```python
from build123d import *

# Parameters (mm, degrees)
SKETCH1_W           = 156
SKETCH1_H           = 90
BOSS_EXTRUDE1_DEPTH = 3
SKETCH2_W           = 156
SKETCH2_H           = 90
SKETCH2_W_2         = 150
SKETCH2_H_2         = 84
BOSS_EXTRUDE2_DEPTH = 48
FILLET1_R           = 1
SKETCH3_W           = 12
SKETCH3_H           = 23
CUT_EXTRUDE2_DEPTH  = 157
SKETCH4_R           = 8.5
CUT_EXTRUDE3_DEPTH  = 10


with BuildPart() as part:
    # Sketch1 → Boss-Extrude1 (new body)
    with BuildSketch(Plane(origin=(0, 0, 0), x_dir=(1, 0, 0), z_dir=(0, 1, 0))):
        with Locations((78, 45)):
            Rectangle(SKETCH1_W, SKETCH1_H)
    extrude(amount=BOSS_EXTRUDE1_DEPTH)

    # Sketch2 → Boss-Extrude2 (add)
    with BuildSketch(Plane(origin=(0, 3, 0), x_dir=(1, 0, 0), z_dir=(0, 1, 0))):
        with Locations((78, 45)):
            Rectangle(SKETCH2_W, SKETCH2_H)
        with Locations((78, 45)):
            Rectangle(SKETCH2_W_2, SKETCH2_H_2, mode=Mode.SUBTRACT)
    extrude(amount=BOSS_EXTRUDE2_DEPTH)

    # Fillet1
    fillet1_edges = [part.edges().sort_by_distance(p)[0] for p in [
        (0, 25.5, -90),
        (156, 25.5, -90),
        (156, 25.5, 0),
        (0, 25.5, 0),
    ]]
    fillet(fillet1_edges, radius=FILLET1_R)

    # Sketch3 → Cut-Extrude2 (cut, through all)
    with BuildSketch(Plane(origin=(156, 0, 0), x_dir=(0, 0, -1), z_dir=(1, 0, 0))):
        with Locations((9, 14.5)):
            Rectangle(SKETCH3_W, SKETCH3_H)
        with Locations((81, 14.5)):
            Rectangle(SKETCH3_W, SKETCH3_H)
    extrude(amount=-CUT_EXTRUDE2_DEPTH, mode=Mode.SUBTRACT)

    # Sketch4 → Cut-Extrude3 (cut)
    with BuildSketch(Plane.ZY):
        with Locations((-59, 40)):
            Circle(SKETCH4_R)
        with Locations((-31, 40)):
            Circle(SKETCH4_R)
    extrude(amount=-CUT_EXTRUDE3_DEPTH, mode=Mode.SUBTRACT)


solid = part.part
```
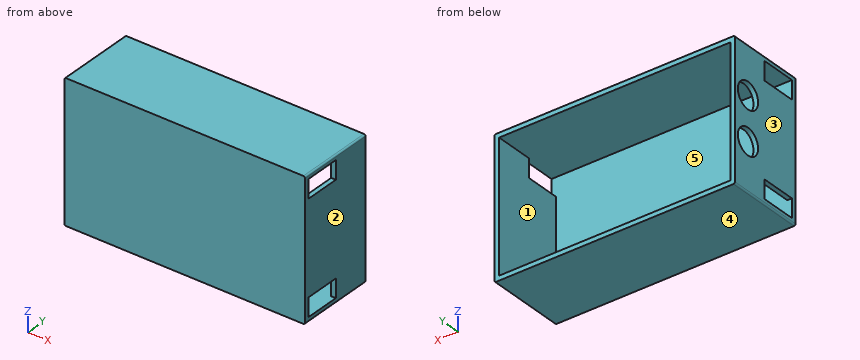
The listing builds one solid part. Answer for the finished solid, in the listing's coordinates (mm). Face numbers are marked on the shaded views. A direction names the side the tool comes from. Give positions to 0.01 mm unless a question says otherwise; leave off trailing zeros. Order: outer loops, then holes, each group sorted by start corner. A loop starts at its lowest first (then second) coordinate and runs counter-clockwise, first axis right, second up. Notation, with made-up numbers: (64.5, -26.75) -> (75.5, -26.75) arc R6 ccw to (75.5, -19.75) -> close; hole circle Ø11 at (-24, 58). An arc over 180 degrees is marked (long way). Answer as a JSON object with one key per item and string values. Group by question number.
Item 1: A tool of negligible diameter and unlimited length cuts with its end or side. For the marked faces 1 and 2, from which of +Z, -Z, +X, -X, +Y, -Y can it reach the whole face along a straight path? Write none if from no direction.
Item 2: Determine the mould class of the marked faces 3, 4 and 5 for opening direction Z: pulls with the +Z half, pulls with the -Z half, needs draft (parallel to the pull), parting line crosses it, or undercut.
Item 3: The part is cut by section B-B on z = -59. Write down the section's boundary in (x, y), and give its area (3 significant figures).
Item 4: Consider L1, parallel to Y at x = 1.3, z = -31; L2, parallel to Z at x = 87.5, y = 31.5; L3, parallel to X at y = 34, z = -15. Determine where each line is inside the solid, lowest interval first. Write a range as from..to.
Item 5: The part is cut by section A-A on y = 6.5. Write down the section's boundary in (x, z), and give its area (3 significant figures).
Item 6: The part is cut by section D-D on z = -78.5. Write down the section's boundary in (x, y), and give its area (3 significant figures).
Item 7: The part is cut by section C-C on y = 40. Write down the section's boundary in (x, z).
Item 8: Flat-ended cylindrical pins translate along their axes: pin 1 (12 mm diameter, centred on x = 131.5, z = -65.5, fed in from +Y); pin 2 (15.5 mm diameter, centred on y = 40, z = -31, fed in from -X). Find the tip coordinate at first contact, or state that the pin passes through.
Result set:
{
 "1": {"face 1": "+Y", "face 2": "+Z, -Z, +X, +Y, -Y"},
 "2": {"face 3": "needs draft", "face 4": "pulls with the -Z half", "face 5": "undercut"},
 "3": {"outline": "(0, 0) -> (156, 0) -> (156, 51) -> (153, 51) -> (153, 3) -> (3, 3) -> (3, 31.5) -> (0, 31.5) -> close; (0, 48.5) -> (3, 48.5) -> (3, 51) -> (0, 51) -> close", "area": "705 mm²"},
 "4": {"L1": "0..31.5, 48.5..51", "L2": "-90..-87, -3..0", "L3": "0..3, 153..156"},
 "5": {"outline": "(0, -89) arc R1 ccw to (1, -90) -> (155, -90) arc R1 ccw to (156, -89) -> (156, -87) -> (0, -87) -> close; (0, -75) -> (3, -75) -> (3, -15) -> (0, -15) -> close; (0, -3) -> (156, -3) -> (156, -1) arc R1 ccw to (155, 0) -> (1, 0) arc R1 ccw to (0, -1) -> close; (153, -75) -> (156, -75) -> (156, -15) -> (153, -15) -> close", "area": "1,300 mm²"},
 "6": {"outline": "(0, 0) -> (156, 0) -> (156, 3) -> (0, 3) -> close; (0, 26) -> (3, 26) -> (3, 51) -> (0, 51) -> close; (153, 26) -> (156, 26) -> (156, 51) -> (153, 51) -> close", "area": "618 mm²"},
 "7": {"outline": "(0, -89) arc R1 ccw to (1, -90) -> (155, -90) arc R1 ccw to (156, -89) -> (156, -1) arc R1 ccw to (155, 0) -> (1, 0) arc R1 ccw to (0, -1) -> (0, -22.5) -> (3, -22.5) -> (3, -3) -> (153, -3) -> (153, -87) -> (3, -87) -> (3, -67.5) -> (0, -67.5) -> close; (0, -50.5) -> (3, -50.5) -> (3, -39.5) -> (0, -39.5) -> close"},
 "8": {"pin 1": "y = 3", "pin 2": "x = 153"}
}
